Could you check a few things on this model? Use its own coordinates, in mm. Face numbers are marked on the shaded views. A direction names the side the tool comes from. Give positions to 0.01 mm unless a question says otherwise; leave off trailing zeros. Loops run counter-clockwise (first coordinate to the right, second up) from the corner with the lowest first, then second, coordinate; pieces in that order, holes last.
1. Imagine slicing it at C-C (z = -1.5). List the corners of the cut face in (x, y) for me, plus the area to 3 significant figures.
2. For P1, Ø2, axis at y = 0, z = -8.5, coming from the +X side; P2, Ø1.5, axis at y = 3, z = 4, coming from the +X side; P3, Ø2, axis at y = 3, z = 0, coming from the -X side, each with a flat end and sliding along its axis, tell me the tip position at first contact or that it passes through.
3. I need wall thicknesses on line 1 along X through (y, z) = (0, 0.5); line 2 along X through (y, z) = (0, -7.5). Which ranges of each line are inside material? Lowest first, please.
4. Imagine slicing it at D-D (y = -1.5). List the corners of the cut face in (x, z) for me, plus the area to 3 significant figures.
5. For the marked faces 1, 2 and 3, which set-ups out of +Z, -Z, +X, -X, +Y, -Y let a thin tool reach every point of the face, with its end or its side?
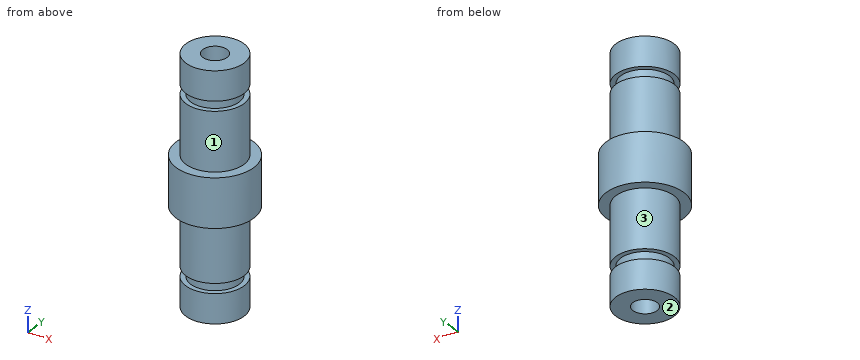
Autodesk Inventor part; units mm, degrees
ref_plane "YZ Plane" through (0, 0, 0) normal (1, 0, 0) x (0, 1, 0)
ref_plane "XZ Plane" through (0, 0, 0) normal (0, 1, 0) x (-1, 0, 0)
ref_plane "XY Plane" through (0, 0, 0) normal (0, 0, 1) x (1, 0, 0)
sketch "スケッチ2" plane through (0, 0, 0) normal (1, 0, 0) x (0, 1, 0)
  line L0 (2.5, -8.5) -> (3, -8.5)
  line L1 (3, -9.5) -> (2.5, -9.5)
  line L2 (2.5, -9.5) -> (2.5, -8.5)
  line L3 (3, -9.5) -> (3, -12.5)
  line L4 (3, -12.5) -> (1.25, -12.5)
  line L5 (1.25, -12.5) -> (1.25, 0)
  line L6 (1.25, 0) -> (4, 0)
  line L7 (4, 0) -> (4, -2.5)
  line L8 (4, -2.5) -> (3, -2.5)
  line L9 (3, -2.5) -> (3, -8.5)
  line L10 (0, -15) -> (0, 2.5)
  point P0 (0, 0)
  dimension "d3" = 8.5
  dimension "d4" = 1
  dimension "d5" = 2.5
  dimension "d6" = 1.25
  dimension "d8" = 4
  dimension "d9" = 2.5
  dimension "d10" = 3
  dimension "d11" = 12.5
revolve "回転1" add sketch "スケッチ2" angle 360 about axis through (0, 0, -10) along (0, 0, 1)
mirror "ミラー1" about plane through (0, 4, 0) normal (0, 0, 1) of "回転1"
sketch "スケッチ1" plane through (0, 0, 0) normal (0, 0, 1) x (1, 0, 0)
  circle A0 centre (0, 0) radius 4
  dimension "d0" = 8
properties part number "下側ベアリング軸" material "アルミニウム 2014-T4"
Derived:
1. outline: circle Ø8 at (0, 0); hole circle Ø2.5 at (0, 0)
1. area: 45.4 mm2
2. P1: stops at x = 3
2. P2: stops at x = 1.98
2. P3: stops at x = -3.46
3. line 1: x = -4 to -1.25, 1.25 to 4
3. line 2: x = -3 to -1.25, 1.25 to 3
4. outline: (-3.71, -2.5) - (-2.6, -2.5) - (-2.6, -8.5) - (-2, -8.5) - (-2, -9.5) - (-2.6, -9.5) - (-2.6, -12.5) - (2.6, -12.5) - (2.6, -9.5) - (2, -9.5) - (2, -8.5) - (2.6, -8.5) - (2.6, -2.5) - (3.71, -2.5) - (3.71, 2.5) - (2.6, 2.5) - (2.6, 8.5) - (2, 8.5) - (2, 9.5) - (2.6, 9.5) - (2.6, 12.5) - (-2.6, 12.5) - (-2.6, 9.5) - (-2, 9.5) - (-2, 8.5) - (-2.6, 8.5) - (-2.6, 2.5) - (-3.71, 2.5) - close
4. area: 139 mm2
5. face 1: +Z
5. face 2: -Z, +X, -X, +Y, -Y
5. face 3: -Z
